```python
from build123d import *

# Parameters (mm, degrees)
SKETCH1_R           = 2.794
SKETCH1_R_2         = 1.212486465
BOSS_EXTRUDE1_DEPTH = 9.144
FILLET1_R           = 0.0762
FILLET2_R           = 1.27
FILLET3_R           = 1.27
FILLET4_R           = 1.27


with BuildPart() as part:
    # Sketch1 → Boss-Extrude1 (new body)
    with BuildSketch(Plane(origin=(0, 0, 0), x_dir=(0, 0, -1), z_dir=(1, 0, 0))):
        with BuildLine():
            Line((7.455728261, -0.746434927), (0, 7.493))
            ThreePointArc((0, 7.493), (-2.216071025, 7.157798419), (-4.23386886, 6.182184362))
            Line((-4.23386886, 6.182184362), (-12.48371449, 18.228392766))
            ThreePointArc((-12.48371449, 18.228392766), (-13.557344424, 18.890595677), (-14.768732641, 18.538839342))
            ThreePointArc((-14.768732641, 18.538839342), (-20.873202748, 14.088773121), (-27.541235985, 10.538424208))
            ThreePointArc((-27.541235985, 10.538424208), (-28.725821969, 8.525909619), (-27.207679666, 6.751451146))
            Line((-27.207679666, 6.751451146), (-7.27244078, 1.804620212))
            ThreePointArc((-7.27244078, 1.804620212), (-5.186520816, -5.407869342), (2.106798928, -7.190719524))
            Line((2.106798928, -7.190719524), (1.642588995, -5.606323697))
            ThreePointArc((1.642588995, -5.606323697), (4.675733574, -3.50235343), (5.842, 0))
            Line((5.842, 0), (7.455728261, -0.746434927))
        make_face()
        Circle(SKETCH1_R, mode=Mode.SUBTRACT)
        with Locations((-26.723594694, 8.702265656)):
            Circle(SKETCH1_R_2, mode=Mode.SUBTRACT)
    extrude(amount=BOSS_EXTRUDE1_DEPTH)

    # Fillet1
    fillet1_edges = [part.edges().sort_by_distance(p)[0] for p in [
        (4.572, -0.746434927, -7.455728261),
    ]]
    fillet(fillet1_edges, radius=FILLET1_R)

    # Fillet2
    fillet2_edges = [part.edges().sort_by_distance(p)[0] for p in [
        (4.572, 6.182184362, 4.23386886),
    ]]
    fillet(fillet2_edges, radius=FILLET2_R)

    # Fillet3
    fillet3_edges = [part.edges().sort_by_distance(p)[0] for p in [
        (4.572, 7.493, 0),
    ]]
    fillet(fillet3_edges, radius=FILLET3_R)

    # Fillet4
    fillet4_edges = [part.edges().sort_by_distance(p)[0] for p in [
        (4.572, 1.804620212, 7.27244078),
    ]]
    fillet(fillet4_edges, radius=FILLET4_R)


solid = part.part
```
Can you work these out from the model? Positions are in its coordinate system, mm. A direction names the side the tool comes from. Round coordinates to 2 decimals unless told otherwise and drop trailing zeros. Loops run counter-clockwise (first coordinate to the right, second up) from the corner with the lowest first, then second, coordinate; pieces in that order, holes last. Notation, with made-up numbers: M -28,52.5 L -9,52.5 A33 ccw -9,81.5 Z; hole C 20,24 d9. An arc over 180 degrees is marked long. Answer in a Markdown table with one row per item.
1. If we section it at D-D, the plane z = -4: Please give me the cut outline in (x, y).
Established:
| item | result |
|---|---|
| outline | M 0,-4.26 L 9.14,-4.26 L 9.14,3.07 L 0,3.07 Z |
2. If we section it at B-B, the plane x = 1.5: Give the number of separate pieces and of enclosed holes in the cut face, plus the area to 3 significant figures.
Established:
| item | result |
|---|---|
| separate pieces | 1 |
| enclosed holes | 2 |
| area | 341 mm² |
3. If we section it at A-A, the plane z = 0: Please give me the cut outline in (x, y).
Established:
| item | result |
|---|---|
| outline | M 0,-7.49 L 9.14,-7.49 L 9.14,-2.79 L 0,-2.79 Z; M 0,2.79 L 9.14,2.79 L 9.14,7.35 L 0,7.35 Z |
4. Thinking about a two-plate mould opening in Y: for faces 1 (the face through (4.636, 7.385, 0.086)), 2 (the face through (0, 6, 11)), 3 (the face through (4.51, -6.41, -1.88)), which applies, pulls with the +Y half, pulls with the -Y half, needs draft (parallel to the pull), parting line crosses it, or undercut?
Established:
| item | result |
|---|---|
| face 1 | pulls with the +Y half |
| face 2 | needs draft |
| face 3 | undercut |
5. If we section it at C-C, the plane y = -3.25: Please give me the cut outline in (x, z).
Established:
| item | result |
|---|---|
| outline | M 0,-4.85 L 9.14,-4.85 L 9.14,6.75 L 0,6.75 Z |
6. On a 3-axis mill with a long thin cutter (end or side, diameter ignored), from which of +Z, -Z, +X, -X, +Y, -Y can I reach the whole of each face in a straight line? I mean faces 4 (the face through (4.51, 7.63, 26.16)), 5 (the face through (4.508, 7.224, 1.988)), 6 (the face through (4.51, -0.29, -6.47)). Say none if no direction works.
Established:
| item | result |
|---|---|
| face 4 | +X, -X |
| face 5 | +X, -X, +Y |
| face 6 | +X, -X, -Y |
7. I'm going to push flat-ended pins straight in: pin 1 Ø1.5 at (x, z) = (2.5, 8.5) entering from +Y; pin 2 Ø5 at (x, y) = (6.5, -1.5) entering from +Z; pin 3 Ø1.5 at (x, z) = (8, 11) entering from -Y. Where does each tip first touch, or does it pass through?
Established:
| item | result |
|---|---|
| pin 1 | y = 13.51 |
| pin 2 | z = 7.49 |
| pin 3 | y = 2.54 |
8. Please list where these lines run through material, in increasing order: line 1 (Y direction, x = 5.25, z = 0); line 2 (Y direction, x = 8.5, z = 2.5); line 3 (Z direction, x = 0.5, y = -2.5). Write a range as from..to.
Established:
| item | result |
|---|---|
| line 1 | -7.49..-2.79, 2.79..7.35 |
| line 2 | -7.06..-1.25, 1.25..7.06 |
| line 3 | -5.28..-1.25, 1.25..7.06 |
